```python
from build123d import *

# Parameters (mm, degrees)
SKETCH1_W           = 3
SKETCH1_H           = 89
BOSS_EXTRUDE1_DEPTH = 0.4
BOSS_EXTRUDE2_DEPTH = 0.5
SKETCH3_W           = 2
SKETCH3_H           = 12
BOSS_EXTRUDE3_DEPTH = 8.6
FILLET1_R           = 2
SKETCH4_R           = 2.1
CUT_EXTRUDE1_DEPTH  = 47.997659516


with BuildPart() as part:
    # Sketch1 → Boss-Extrude1 (new body)
    with BuildSketch(Plane(origin=(0, 0, 0), x_dir=(1, 0, 0), z_dir=(0, 1, 0))):
        Rectangle(SKETCH1_W, SKETCH1_H)
    extrude(amount=BOSS_EXTRUDE1_DEPTH)

    # Sketch2 → Boss-Extrude2 (add)
    with BuildSketch(Plane(origin=(0, 0.4, 0), x_dir=(1, 0, 0), z_dir=(0, 1, 0))):
        Polygon((3, 9.5), (3, 44.5), (-3, 44.5), (-3, -44.5), (3, -44.5), (3, -2.5), (9.7, -2.5), (9.7, 9.5), align=None)
    extrude(amount=BOSS_EXTRUDE2_DEPTH)

    # Sketch3 → Boss-Extrude3 (add)
    with BuildSketch(Plane.XZ.offset(-0.4)):
        with Locations((8.7, -3.5)):
            Rectangle(SKETCH3_W, SKETCH3_H)
    extrude(amount=BOSS_EXTRUDE3_DEPTH)

    # Fillet1
    fillet1_edges = [part.edges().sort_by_distance(p)[0] for p in [
        (9.7, -3.65, 2.5),
        (9.7, -3.65, -9.5),
    ]]
    fillet(fillet1_edges, radius=FILLET1_R - 0.0001)  # a hair under: the kernel refuses the full size

    # Sketch4 → Cut-Extrude1 (cut, through all)
    with BuildSketch(Plane(origin=(9.7, 0, 0), x_dir=(0, 0, -1), z_dir=(1, 0, 0))):
        with Locations((3.5, -2.6)):
            Circle(SKETCH4_R)
    extrude(amount=-CUT_EXTRUDE1_DEPTH, mode=Mode.SUBTRACT)


solid = part.part
```
The model under review builds one solid part; all positions refer to its coordinate system, in mm. A direction names the side the tool comes from. Round coordinates to 2 decimals unless told otherwise and drop trailing zeros. Loops run counter-clockwise (first coordinate to the right, second up) from the corner with the lowest first, then second, coordinate; pieces in that order, holes last. Notation, with made-up numbers: M 53,-6.75 L 89,-6.75 A24 cw 89,3.25 Z; hole C 39,7.25 d2. An arc over 180 degrees is marked long. Put each result on its own line as item: value.
Q1. Mouldability with a two-part tool opening along Y and no side actions: class faces 1 (the cylindrical face through (9.13, -3.71, -8.9)), 2 (the cylindrical face through (8.714, -1.969, -5.503)), 3 (the flat face through (0, 0, -1)) as released by +Y, released by -Y, zero draft, split by the parting line, or undercut.
Result set:
face 1: zero draft
face 2: undercut
face 3: released by -Y
Q2. Machinability: for faces 4 (the flat face through (9.7, -5, -4)), 5 (the flat face through (3, 0.4, 0)), 6 (the flat face through (-2, 0.4, -1)), 7 (the flat face through (5.34, 0.75, -9.5)), 8 (the flat face through (5.34, 0.75, 2.5)), which of the approach directions +Z, -Z, +X, -X, +Y, -Y give a long, thin tool a straight path to every point of the face, cutting with its end or side? Answer none if there is none.
Result set:
face 4: +Z, -Z, +X, +Y, -Y
face 5: +Z, -Z, -Y
face 6: +Z, -Z, -X, -Y
face 7: -Z, +X, +Y, -Y
face 8: +Z, +X, +Y, -Y
Q3. To check wall thickness, follow L1, parallel to Y at x = 8.75, z = -3.5; L2, parallel to Y at x = -2, z = -39.5; L3, parallel to X at y = -4.25, z = 0.5. State the ranges of each line that lie inside material, in increasing order.
Result set:
L1: y = -8.2 to -4.7, -0.5 to 0.9
L2: y = 0.4 to 0.9
L3: x = 7.7 to 9.7
Q4. Consider section C-C, the plane z = 39. Give the boundary of the cut face in (x, y), then the cut area to 3 significant figures.
Result set:
outline: M -3,0.4 L -1.5,0.4 L -1.5,0 L 1.5,0 L 1.5,0.4 L 3,0.4 L 3,0.9 L -3,0.9 Z
area: 4.20 mm²
Q5. Consider section A-A, the plane z = -3.5. Give the boundary of the cut face in (x, y), then the cut area to 4 significant figures.
Result set:
outline: M -3,0.4 L -1.5,0.4 L -1.5,0 L 1.5,0 L 1.5,0.4 L 7.7,0.4 L 7.7,-0.5 L 9.7,-0.5 L 9.7,0.9 L -3,0.9 Z; M 7.7,-8.2 L 9.7,-8.2 L 9.7,-4.7 L 7.7,-4.7 Z
area: 16.35 mm²
Q6. For pin 1 (4 mm diameter, centred on x = 8, y = -6.5, fed in from -Z); pin 2 (1.6 mm diameter, centred on x = -2, z = 17.5, fed in from -Y); pin 3 (4 mm diameter, centred on x = 4, z = -27.5, fed in from -Y), all flat-tipped, find the tip position at first contact; note any pin that passes through.
Result set:
pin 1: stops at z = -9.5
pin 2: stops at y = 0
pin 3: stops at y = 0.4
Q7. Consider section D-D, the plane x = -0.5. Give the boundary of the cut face in (y, z).
Result set:
outline: M 0,-44.5 L 0.9,-44.5 L 0.9,44.5 L 0,44.5 Z
